```python
from build123d import *

# Parameters (mm, degrees)
F0_W      = 200
F0_H      = 200
F1_DEPTH  = 120
F2_W      = 110
F2_H      = 76.8
F2_H_2    = 113.2
F3_DEPTH  = 200
F5_R      = 4.25
F6_DEPTH  = 10
F7_R      = 4.25
F8_DEPTH  = 10
F9_R      = 4.25
F10_DEPTH = 10


with BuildPart() as f1:
    # F0 (on Front) → F1 (new body)
    with BuildSketch(Plane.XZ):
        Rectangle(F0_W, F0_H)
    extrude(amount=F1_DEPTH)

    # F2 (on face) → F3 (cut)
    with BuildSketch(Plane.YZ.offset(100)):
        with Locations((-55, 61.6)):
            Rectangle(F2_W, F2_H)
        with Locations((-55, -43.4)):
            Rectangle(F2_W, F2_H_2)
    extrude(amount=-F3_DEPTH, mode=Mode.SUBTRACT)

    # F5 (on face) → F6 (cut)
    with BuildSketch(Plane(origin=(0, -110, 0), x_dir=(-1, 0, 0), z_dir=(0, 1, 0))):
        with Locations((-85, 85)):
            Circle(F5_R)
        with Locations((85, 85)):
            Circle(F5_R)
    extrude(amount=-F6_DEPTH, mode=Mode.SUBTRACT)

    # F7 (on face) → F8 (cut)
    with BuildSketch(Plane(origin=(0, -110, 0), x_dir=(-1, 0, 0), z_dir=(0, 1, 0))):
        with Locations((-85, -85)):
            Circle(F7_R)
    extrude(amount=-F8_DEPTH, mode=Mode.SUBTRACT)

    # F9 (on face) → F10 (cut)
    with BuildSketch(Plane(origin=(0, -110, 0), x_dir=(-1, 0, 0), z_dir=(0, 1, 0))):
        with Locations((85, -85)):
            Circle(F9_R)
    extrude(amount=-F10_DEPTH, mode=Mode.SUBTRACT)


solid = f1.part
```
CAD build for the part. Positions are in the model's coordinates, mm. A direction names the side the tool comes from. Round coordinates to 2 decimals unless told otherwise and drop trailing zeros. Order: outer loops, then holes, each group sorted by start corner. A loop starts at its lowest first (then second) coordinate and runs counter-clockwise, first axis right, second up.
Item 1: Saw through at D-D on y = -105.5. Write the cut outline in (x, z), then the cut area to 3 significant figures.
Item 2: Probe line 1 along Z through (x, y) = (85, -115); line 2 along X through (y, z) = (-111.5, -86.5); line 3 along Y through (x, z) = (65, -87). List the from-to ranges inside material, lowest first.
Item 3: Saw through at B-B on x = -85. Write the cut outline in (y, z).
Item 4: Saw through at A-A on z = -85. Write the cut outline in (x, y).
Item 5: Mould opens along X. For faces 1 (the face through (-1, -115, 100)), 2 (the face through (-84.08, -114.93, -89.15)), 3 (the face through (100, -86, 14)), 4 (the face through (-100, -86, 14)) say: pulls with the +X half, pulls with the -X half, needs draft (parallel to the pull), parting line crosses it, or undercut.
Item 6: Tool access for faces 5 (the face through (1, -110, -44)), 6 (the face through (-1, 0, 18)), 7 (the face through (1, -56, 23.2)): list every direction of +Z, -Z, +X, -X, +Y, -Y with a clear straight run to the whole face (end or side of a thin tool).
Item 7: Pin check, flat tips, straight feed: pin 1 (6 mm diameter, centred on x = -42, y = -56.5, fed in from -Z); pin 2 (1.5 mm diameter, centred on x = 62.5, y = -66, fed in from +Z); pin 3 (10 mm diameter, centred on x = 85, z = 85, fed in from +Y). Stop position of each tip, or through.
Item 8: Saw through at C-C on x = 42. Write the cut outline in (y, z), then the cut area to 3 significant figures.
Reported:
1. outline: (-100, 13.2) - (100, 13.2) - (100, 23.2) - (-100, 23.2) - close
1. area: 2,000 mm2
2. line 1: z = -100 to -89.25, -80.75 to 80.75, 89.25 to 100
2. line 2: x = -100 to -88.98, -81.02 to 81.02, 88.98 to 100
2. line 3: y = -120 to -110
3. outline: (-120, -100) - (-110, -100) - (-110, -89.25) - (-120, -89.25) - close; (-120, -80.75) - (-110, -80.75) - (-110, 13.2) - (0, 13.2) - (0, 23.2) - (-110, 23.2) - (-110, 80.75) - (-120, 80.75) - close; (-120, 89.25) - (-110, 89.25) - (-110, 100) - (-120, 100) - close
4. outline: (-100, -120) - (-89.25, -120) - (-89.25, -110) - (-100, -110) - close; (-80.75, -120) - (80.75, -120) - (80.75, -110) - (-80.75, -110) - close; (89.25, -120) - (100, -120) - (100, -110) - (89.25, -110) - close
5. face 1: needs draft
5. face 2: undercut
5. face 3: pulls with the +X half
5. face 4: pulls with the -X half
6. face 5: -Z, +X, -X, +Y
6. face 6: +Z, -Z, +X, -X, +Y
6. face 7: +Z, +X, -X, +Y
7. pin 1: stops at z = 13.2
7. pin 2: stops at z = 23.2
7. pin 3: stops at y = -110
8. outline: (-120, -100) - (-110, -100) - (-110, 13.2) - (0, 13.2) - (0, 23.2) - (-110, 23.2) - (-110, 100) - (-120, 100) - close
8. area: 3,100 mm2
